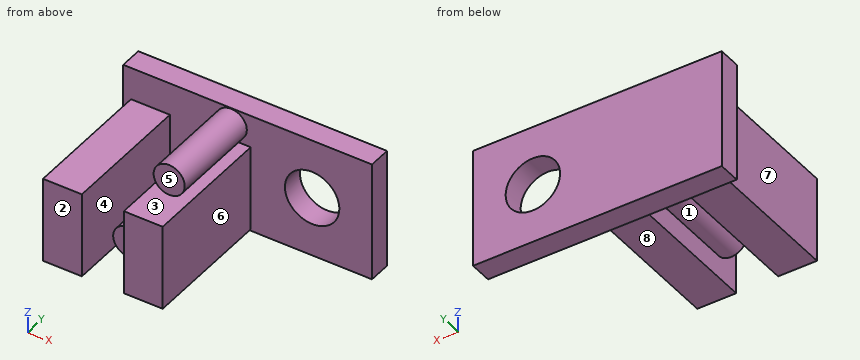
Autodesk Inventor part; units mm, degrees
ref_plane "YZ Plane" through (0, 0, 0) normal (1, 0, 0) x (0, 1, 0)
ref_plane "XZ Plane" through (0, 0, 0) normal (0, 1, 0) x (-1, 0, 0)
ref_plane "XY Plane" through (0, 0, 0) normal (0, 0, 1) x (1, 0, 0)
sketch "Náčrt1" plane through (0, 0, 0) normal (0, 1, 0) x (-1, 0, 0)
  line L0 (8, -3.85) -> (-8, -3.85)
  line L1 (-8, -3.85) -> (-8, 3.85)
  line L2 (-8, 3.85) -> (8, 3.85)
  line L3 (8, 3.85) -> (8, -3.85)
  line L4 (8, -3.85) -> (0, 0) construction
  line L5 (8, 3.85) -> (0, 0) construction
  line L6 (-8, -3.85) -> (0, 0) construction
  dimension "d0" = 16
  dimension "d1" = 7.7
extrude "Vysunutí1" add sketch "Náčrt1" along normal blind 1.45
sketch "Náčrt2" plane through (0, 0, 0) normal (0, -1, 0) x (1, 0, 0)
  line L0 (0.2, 1.75) -> (-2.3, 1.75)
  line L1 (-2.3, 1.75) -> (-2.3, -3.75)
  line L2 (-2.3, -3.75) -> (0.2, -3.75)
  line L3 (0.2, -3.75) -> (0.2, 1.75)
  line L4 (-5, 1.75) -> (-7.5, 1.75)
  line L5 (-7.5, 1.75) -> (-7.5, -3.75)
  line L6 (-7.5, -3.75) -> (-5, -3.75)
  line L7 (-5, -3.75) -> (-5, 1.75)
  line L8 (-8, -3.85) -> (-8, 3.85)
  line L9 (-2.3, 1.75) -> (-5, 1.75) construction
  circle A0 centre (-3.65, -2.45) radius 1
  circle A1 centre (-1.05, 2.8) radius 1
  line L10 (-1.05, 1.75) -> (-1.05, 2.8) construction
  line L11 (-1.05, 2.8) -> (-1.05, 3.85) construction
  line L12 (-2.3, -2.45) -> (-3.65, -2.45) construction
  line L13 (-3.65, -2.45) -> (-5, -2.45) construction
  line L14 (-3.65, 1.75) -> (-3.65, 0.35) construction
  line L15 (-3.65, 0.35) -> (-3.65, -1.05) construction
  line L16 (-3.65, -1.05) -> (-3.65, -2.45) construction
  line L17 (-3.65, -3.85) -> (-3.65, -2.45) construction
  point P0 (0, 0)
  dimension "d4" = 2.5
  dimension "d5" = 5.5
  dimension "d6" = 0.5
  dimension "d7" = 2
  dimension "d8" = 2.7
  dimension "d15" = 0.1
extrude "Vysunutí2" add sketch "Náčrt2" along normal blind 8.5 contours L3 L2 L1 L0 | L7 L6 L5 L4
extrude "Vysunutí3" add sketch "Náčrt2" along normal blind 6 contours A0 | A1
sketch "Náčrt3" plane through (0, 1.45, 0) normal (0, 1, 0) x (1, 0, 0)
  line L0 (8, -3.85) -> (8, 3.85)
  line L1 (8, -3.85) -> (4.15, -3.85)
  line L2 (4.15, -3.85) -> (4.15, 0)
  line L3 (4.15, 0) -> (8, 0)
  line L4 (8, 0) -> (8, -3.85)
  line L5 (8, 3.85) -> (-8, 3.85)
  line L6 (8, 3.85) -> (4.15, 3.85)
  line L7 (4.15, 3.85) -> (4.15, 0)
  line L8 (4.15, 0) -> (8, 0)
  line L9 (8, 0) -> (8, 3.85)
  point P0 (0, 0)
hole "Díra1" at (4.15, 1.45, 0) direction (0, -1, 0) diameter 3.5 end through all
properties part number "qre_module"
Read the model definition and answer for the solid it produces. Units are mm, in the model's axes. Face numbers are marked on the shaded views. A direction names the side the tool comes from. Give positions to 0.01 mm unless a question says otherwise; leave off trailing zeros. Write each loop counter-clockwise with the first axis right and the second up, starting at its lowest first coordinate (ties: lowest second). Pieces come first, ordered by that corner, then holes. Notation, with made-up numbers: (39.25, 76.25) - (94.25, 76.25) arc R6 cw to (94.25, 84.25) - close; hole circle Ø11 at (36, 31). An arc over 180 degrees is marked (long way). Use CSV: the item, a comma, the result in double quotes. Start each with the question number.
Item 1: The part is cut by section D-D, the plane y = -5.25. Give the vertices of the cut face in (x, z).
Item 2: The part is cut by section A-A, the plane x = 4.15. Give the vertices of the cut face in (y, z), and give its area (3 significant figures).
Item 3: Consider line 1 (X direction, y = 1.05, z = 0); line 2 (X direction, y = -5, z = -0.5); line 3 (X direction, y = -4.5, z = -2.25). Determine where each line is inside the solid, lowest interval first.
Item 4: The mould has two halves that part along Z. Classify the marked faces 1, 2 and 3: pulls with the +Z half, pulls with the -Z half, needs draft (parallel to the pull), parting line crosses it, or undercut.
Item 5: Flat-ended cylindrical pins translate along their axes: P1, Ø1.6, axis at y = -3.5, z = -1, coming from the -X side; P2, Ø2, axis at x = -1.5, y = -2.5, coming from the -Z side; P3, Ø1.6, axis at x = -4, z = -2, coming from the -Y side. Find the tip coordinate at first contact, or state that the pin passes through.
Item 6: The part is cut by section B-B, the plane y = -6.5. Give the vertices of the cut face in (x, z), and give its area (3 significant figures).
Item 7: The part is cut by section C-C, the plane z = 0. Give the vertices of the cut face in (x, y).
Item 8: For the marked faces 4, 5, 6, 7 and 8, determine the directions among +Z, -Z, +X, -X, +Y, -Y from which every point of the face is accessible in a straight line to the end or side of a thin tool.
Taken from the geometry:
1,outline,"(-7.5, -3.75) - (-5, -3.75) - (-5, 1.75) - (-7.5, 1.75) - close; circle Ø2 at (-3.65, -2.45); (-2.3, -3.75) - (0.2, -3.75) - (0.2, 1.75) - (-2.3, 1.75) - close; circle Ø2 at (-1.05, 2.8)"
2,outline,"(0, -3.85) - (1.45, -3.85) - (1.45, -1.75) - (0, -1.75) - close; (0, 1.75) - (1.45, 1.75) - (1.45, 3.85) - (0, 3.85) - close"
2,area,"6.09 mm2"
3,line 1,"-8 to 2.4, 5.9 to 8"
3,line 2,"-7.5 to -5, -2.3 to 0.2"
3,line 3,"-7.5 to -5, -4.63 to -2.67, -2.3 to 0.2"
4,face 1,"parting line crosses it"
4,face 2,"needs draft"
4,face 3,"undercut"
5,P1,"x = -7.5"
5,P2,"z = -3.75"
5,P3,"y = -6"
6,outline,"(-7.5, -3.75) - (-5, -3.75) - (-5, 1.75) - (-7.5, 1.75) - close; (-2.3, -3.75) - (0.2, -3.75) - (0.2, 1.75) - (-2.3, 1.75) - close"
6,area,"27.5 mm2"
7,outline,"(-8, 0) - (-7.5, 0) - (-7.5, -8.5) - (-5, -8.5) - (-5, 0) - (-2.3, 0) - (-2.3, -8.5) - (0.2, -8.5) - (0.2, 0) - (2.4, 0) - (2.4, 1.45) - (-8, 1.45) - close; (5.9, 0) - (8, 0) - (8, 1.45) - (5.9, 1.45) - close"
8,face 4,"+Z, -Z, -Y"
8,face 5,"+Z, +X, -X, -Y"
8,face 6,"+Z, -Z, +X, -Y"
8,face 7,"+Z, -Z, -X, -Y"
8,face 8,"-Z, +X, -X, -Y"
